Here's the drawing with two shaded views (mm, measured from the low corner). I have some questions. A direction names the side the tool comes from. Coordinates: 2 decimals unless noted, no trailing zeros. Write each loop counter-clockwise with the first axis right and the second up, starting at its lowest first coordinate (ties: lowest second). Pieces come first, ordered by that corner, then holes. Notation, with made-up numbers: (56.25, 55) -> (78.25, 55) arc R21 cw to (78.25, 93) -> close; hole circle Ø10 at (48, -39). An arc over 180 degrees is marked (long way). Put each result on its own line as item: value.
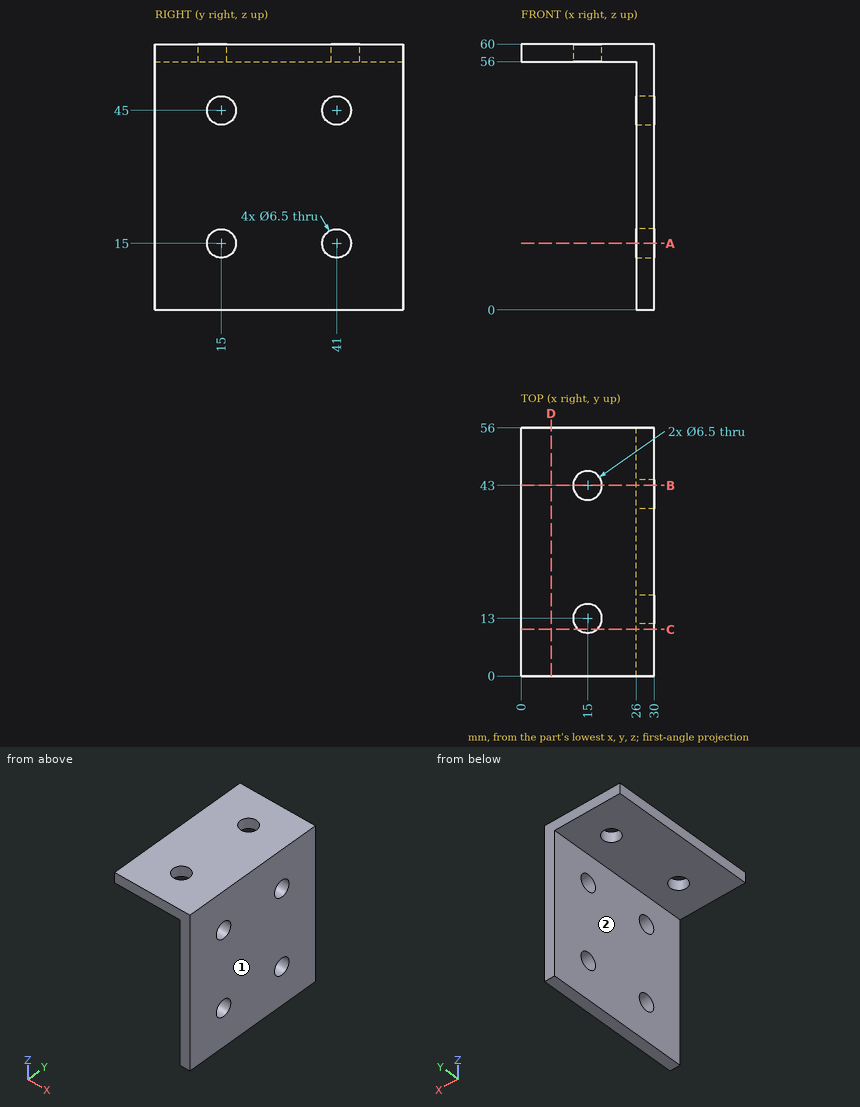
Item 1: Imagine slicing it at D-D on x = 6.75. Write out the boundary of the cut face in (y, z), then the cut area to 3 significant figures.
Output:
outline: (0, 56) -> (56, 56) -> (56, 60) -> (0, 60) -> close
area: 224 mm²
Item 2: For P1, Ø13, axis at x = 18, y = 27, coming from the -Z side; P2, Ø7.5, axis at y = 15, z = 15, coming from the -X side, each with a flat end and sliding along its axis, tell me the tip position at first contact or that it passes through.
Output:
P1: stops at z = 56
P2: stops at x = 26
Item 3: Imagine slicing it at B-B on y = 43. Write out the boundary of the cut face in (x, z), then the cut area to 3 significant figures.
Output:
outline: (0, 56) -> (11.75, 56) -> (11.75, 60) -> (0, 60) -> close; (18.25, 56) -> (26, 56) -> (26, 47.56) -> (30, 47.56) -> (30, 60) -> (18.25, 60) -> close; (26, 0) -> (30, 0) -> (30, 12.44) -> (26, 12.44) -> close; (26, 17.56) -> (30, 17.56) -> (30, 42.44) -> (26, 42.44) -> close
area: 277 mm²
Item 4: Which directions (+Z, -Z, +X, -X, +Y, -Y) give clear straight access to the entire face, cutting with the end or side of a thin tool? Please do the marked faces 1 and 2.
Output:
face 1: +Z, -Z, +X, +Y, -Y
face 2: -Z, -X, +Y, -Y
Item 5: Imagine slicing it at A-A on z = 15. Write out the boundary of the cut face in (x, y).
Output:
outline: (26, 0) -> (30, 0) -> (30, 11.75) -> (26, 11.75) -> close; (26, 18.25) -> (30, 18.25) -> (30, 37.75) -> (26, 37.75) -> close; (26, 44.25) -> (30, 44.25) -> (30, 56) -> (26, 56) -> close
Item 6: Imagine slicing it at C-C on y = 10.5. Write out the boundary of the cut face in (x, z).
Output:
outline: (0, 56) -> (12.92, 56) -> (12.92, 60) -> (0, 60) -> close; (17.08, 56) -> (26, 56) -> (26, 0) -> (30, 0) -> (30, 60) -> (17.08, 60) -> close
Item 7: Please list where these lines run through material, in increasing order: line 1 along Y through (x, z) = (28.75, 15); line 2 along Z through (x, y) = (28.8, 15); line 3 along Y through (x, z) = (15, 59). Write a range as from..to.
Output:
line 1: y = 0..11.75, 18.25..37.75, 44.25..56
line 2: z = 0..11.75, 18.25..41.75, 48.25..60
line 3: y = 0..9.75, 16.25..39.75, 46.25..56
